Solid Edge part; units mm, degrees
sketch "Sketch1" plane through (0, 0, 0) normal (0, 0, 1) x (1, 0, 0)
  line L0 (0, 27) -> (20, 27)
  line L1 (20, 27) -> (20, 24)
  line L2 (13.1, 22.6) -> (20, 24)
  line L3 (13.1, 16.4) -> (20, 15)
  line L4 (20, 15) -> (20, 12)
  line L5 (13.1, 10.6) -> (20, 12)
  line L6 (13.1, 4.4) -> (20, 3)
  line L7 (20, 3) -> (20, 0)
  line L8 (20, 0) -> (0, 0)
  line L9 (0, 0) -> (0, 27)
  arc A0 (13.1, 16.4) -> (13.1, 22.6) centre (13.1, 19.5) cw
  arc A1 (13.1, 4.4) -> (13.1, 10.6) centre (13.1, 7.5) cw
revolve "RevolvedProtrusion1" add sketch "Sketch1" angle 360 about axis through (0, 0, 0) along (0, 1, 0)
sketch "Sketch2" plane through (0, 27, 0) normal (0, 1, 0) x (1, 0, 0)
  line L0 (3.8386, 6.2993) -> (-3.3146, 6.5901)
  arc A0 (-3.3146, 6.5901) -> (-3.536, 6.474) centre (-3.3248, 6.3403) ccw
  line L1 (-3.536, 6.474) -> (-7.3645, 0.4245)
  arc A1 (-7.3645, 0.4245) -> (-7.3746, 0.1747) centre (-7.1532, 0.2908) ccw
  line L2 (-7.3746, 0.1747) -> (-4.0499, -6.1656)
  arc A2 (-3.8386, -6.2993) -> (-4.0499, -6.1656) centre (-3.8285, -6.0495) cw
  line L3 (-3.8386, -6.2993) -> (3.3146, -6.5901)
  arc A3 (3.3146, -6.5901) -> (3.536, -6.474) centre (3.3248, -6.3403) ccw
  line L4 (3.536, -6.474) -> (7.3645, -0.4245)
  arc A4 (7.3645, -0.4245) -> (7.3746, -0.1747) centre (7.1532, -0.2908) ccw
  line L5 (7.3746, -0.1747) -> (4.0499, 6.1656)
  arc A5 (4.0499, 6.1656) -> (3.8386, 6.2993) centre (3.8285, 6.0495) ccw
extrude "Cutout1" cut sketch "Sketch2" along normal through all and the other way through all
properties part number "BumbleB0507"
Work out the finished part from the listing and answer in its coordinate system (mm). A direction names the side the tool comes from. Give positions to 0.01 mm unless a question says otherwise; leave off trailing zeros. Write each loop counter-clockwise with the first axis right and the second up, starting at its lowest first coordinate (ties: lowest second). Pieces come first, ordered by that corner, then holes.
(1) The part is cut by section C-C on z = -17. Count the separate pieces of the cut face and the enclosed holes in it, plus the area to 3 significant figures.
Final values:
separate pieces: 3
enclosed holes: 0
area: 223 mm2
(2) Flat-ended cylindrical pins translate along their axes: pin 1 Ø2 at (x, z) = (-14.5, -12.5) entering from -Y; pin 2 Ø8 at (x, y) = (-13.5, 10.5) entering from -Z; pin 3 Ø5 at (x, y) = (10, 19.5) entering from +Z; pin 4 Ø8 at (y, z) = (14.5, -7) entering from -X. Find the tip coordinate at first contact, or state that the pin passes through.
Final values:
pin 1: stops at y = 0
pin 2: stops at z = -17.44
pin 3: stops at z = 6.63
pin 4: stops at x = -19.77
(3) Which of the six approach directions +Z, -Z, +X, -X, +Y, -Y give full straight-line access (tool end or side, diameter ignored) to faces 1 (the conical face through (-2.933, 16.312, -13.21)), 2 (the flat face through (-5, 27, -5)), 3 (the flat face through (-0.312, 13.311, 6.443))?
Final values:
face 1: none
face 2: +Z, -Z, +X, -X, +Y
face 3: +Y, -Y
(4) The part is cut by section A-A on y = 13.5. Write down the section's boundary in (x, z), plus the area to 3 significant figures.
Final values:
outline: circle Ø40 at (0, 0); hole (-7.37, -0.17) arc R0.25 ccw to (-7.36, -0.42) - (-3.54, -6.47) arc R0.25 ccw to (-3.31, -6.59) - (3.84, -6.3) arc R0.25 ccw to (4.05, -6.17) - (7.37, 0.17) arc R0.25 ccw to (7.36, 0.42) - (3.54, 6.47) arc R0.25 ccw to (3.31, 6.59) - (-3.84, 6.3) arc R0.25 ccw to (-4.05, 6.17) - close
area: 1,110 mm2
(5) The part is cut by section B-B on x = 0. Write down the section's boundary in (y, z), plus the area to 3 significant figures.
Final values:
outline: (0, -20) - (3, -20) - (4.4, -13.1) arc R3.1 cw to (10.6, -13.1) - (12, -20) - (15, -20) - (16.4, -13.1) arc R3.1 cw to (22.6, -13.1) - (24, -20) - (27, -20) - (27, -6.46) - (0, -6.46) - close; (0, 6.46) - (27, 6.46) - (27, 20) - (24, 20) - (22.6, 13.1) arc R3.1 cw to (16.4, 13.1) - (15, 20) - (12, 20) - (10.6, 13.1) arc R3.1 cw to (4.4, 13.1) - (3, 20) - (0, 20) - close
area: 461 mm2
(6) The part is cut by section D-D on y = 5.75. Write down the section's boundary in (x, z).
Final values:
outline: circle Ø21.08 at (0, 0); hole (-7.37, -0.17) arc R0.25 ccw to (-7.36, -0.42) - (-3.54, -6.47) arc R0.25 ccw to (-3.31, -6.59) - (3.84, -6.3) arc R0.25 ccw to (4.05, -6.17) - (7.37, 0.17) arc R0.25 ccw to (7.36, 0.42) - (3.54, 6.47) arc R0.25 ccw to (3.31, 6.59) - (-3.84, 6.3) arc R0.25 ccw to (-4.05, 6.17) - close
(7) The mould has two halves that part along X. Classify faces 4 (the conical face through (-2.933, 4.312, -13.21)), 5 (the flat face through (-5, 0, -5)), 6 (the flat face through (-5.736, 13.311, 2.951)): pulls with the +X half, pulls with the -X half, needs draft (parallel to the pull), parting line crosses it, or undercut.
Final values:
face 4: parting line crosses it
face 5: needs draft
face 6: undercut
(8) Straight lines are drawn through the part: line 1 (Y direction, x = -7.5, z = 7); line 2 (Y direction, x = 0.5, z = -15.5); line 3 (Z direction, x = -1.5, y = 22). For each, find the intervals that lie inside material, in ascending order.
Final values:
line 1: y = 0 to 6.26, 8.74 to 18.26, 20.74 to 27
line 2: y = 0 to 3.91, 11.09 to 15.91, 23.09 to 27
line 3: z = -11.17 to -6.52, 6.39 to 11.17
